Check sheet for the modelled part. Datum: model origin and axes. Units: mm. A direction names the side the tool comes from. Give positions to 0.01 mm unless a question says otherwise; leave off trailing zeros. Order: outer loops, then holes, each group sorted by start corner. A loop starts at its lowest first (then second) coordinate and runs counter-clockwise, first axis right, second up.
```python
from build123d import *

# Parameters (mm, degrees)
SKETCH1_W           = 45.833760325
SKETCH1_H           = 30.125125166
SKETCH1_W_2         = 13.763297708
SKETCH1_H_2         = 9.6
BOSS_EXTRUDE1_DEPTH = 10
SKETCH2_W           = 44.896748031
SKETCH2_H           = 29.260196601
SKETCH2_W_2         = 12.87697359
SKETCH2_H_2         = 10
CUT_EXTRUDE1_DEPTH  = 9


with BuildPart() as part:
    # Sketch1 → Boss-Extrude1 (new body)
    with BuildSketch(Plane.XY):
        with Locations((164.06406709, 6.50813998)):
            Rectangle(SKETCH1_W, SKETCH1_H)
        with Locations((164.223693767, -13.354422603)):
            Rectangle(SKETCH1_W_2, SKETCH1_H_2)
    extrude(amount=BOSS_EXTRUDE1_DEPTH)

    # Sketch2 → Cut-Extrude1 (cut)
    with BuildSketch(Plane.XY.offset(10)):
        with Locations((164.028585862, 6.475675697)):
            Rectangle(SKETCH2_W, SKETCH2_H)
        with Locations((164.12441469, -13.154422603)):
            Rectangle(SKETCH2_W_2, SKETCH2_H_2)
    extrude(amount=-CUT_EXTRUDE1_DEPTH, mode=Mode.SUBTRACT)


solid = part.part
```
Q1. Material ranges on line 1 (Y direction, x = 174, z = 5.5); line 2 (X direction, y = -3, z = 1.5); line 3 (X direction, y = -10, z = 4.5), recorded low to high.
Q2. Sectioned sample at C-C, the plane z = 5.75. Record the cut outline in (x, y).
Q3. Go/stop test with flat-tipped pins: P1, Ø3, axis at y = -11, z = 5, coming from the -X side; P2, Ø10, axis at x = 158, y = -3, coming from the -Z side; P3, Ø6, axis at x = 166, y = -2, coming from the +Z side; P4, Ø3, axis at y = -13, z = 3.5, coming from the +X side. Record where each tip stops, or that it passes through.
Q4. Draft check along Y on faces 1 (the flat face through (179, -8.554, 5)), 2 (the flat face through (164, 6, 0)), 3 (the flat face through (141.58, 6, 6)). Enter one of: pulls with the +Y half, pulls with the -Y half, needs draft (parallel to the pull), parting line crosses it, or undercut.
Q5. Tool access check on faces 4 (the flat face through (149, -8.554, 5)), 5 (the flat face through (178, -8.154, 6)), 6 (the flat face through (157.686, -13, 6)), 7 (the flat face through (171.105, -13, 5)). Record the directions out of +Z, -Z, +X, -X, +Y, -Y that give a thin tool (end or side, any length) a straight path to the whole face; none if there is none.
Q6. Sectioned sample at B-B, the plane x = 155. Record the cut outline in (y, z), plus the area to 3 significant figures.
Q7. Sectioned sample at D-D, the plane x = 161. Record the cut outline in (y, z).
Q8. Sectioned sample at A-A, the plane y = -2. Record the cut outline in (x, z), plus the area to 3 significant figures.
Filled in:
1. line 1: y = -8.55 to -8.15, 21.11 to 21.57
1. line 2: x = 141.15 to 141.58, 186.48 to 186.98
1. line 3: x = 157.34 to 157.69, 170.56 to 171.11
2. outline: (141.15, -8.55) - (157.34, -8.55) - (157.34, -18.15) - (157.69, -18.15) - (157.69, -8.15) - (141.58, -8.15) - (141.58, 21.11) - (186.48, 21.11) - (186.48, -8.15) - (170.56, -8.15) - (170.56, -18.15) - (171.11, -18.15) - (171.11, -8.55) - (186.98, -8.55) - (186.98, 21.57) - (141.15, 21.57) - close
3. P1: stops at x = 157.34
3. P2: stops at z = 0
3. P3: stops at z = 1
3. P4: stops at x = 171.11
4. face 1: pulls with the -Y half
4. face 2: needs draft
4. face 3: undercut
5. face 4: +Z, -Z, -X, -Y
5. face 5: +Z
5. face 6: +Z, -Y
5. face 7: +Z, -Z, +X, -Y
6. outline: (-8.55, 0) - (21.57, 0) - (21.57, 10) - (21.11, 10) - (21.11, 1) - (-8.15, 1) - (-8.15, 10) - (-8.55, 10) - close
6. area: 37.9 mm2
7. outline: (-18.15, 0) - (21.57, 0) - (21.57, 10) - (21.11, 10) - (21.11, 1) - (-18.15, 1) - close
8. outline: (141.15, 0) - (186.98, 0) - (186.98, 10) - (186.48, 10) - (186.48, 1) - (141.58, 1) - (141.58, 10) - (141.15, 10) - close
8. area: 54.3 mm2
